from build123d import *

# Parameters (mm, degrees)
SKETCH_1_R      = 10
SKETCH_1_R_2    = 1.25
SKETCH_1_R_3    = 3
EXTRUDE_1_DEPTH = 2
SKETCH_2_R      = 4.5
SKETCH_2_R_2    = 3
EXTRUDE_2_DEPTH = 1


with BuildPart() as part:
    # 草图1 → 凸台-拉伸1 (new body)
    with BuildSketch(Plane.XY):
        Circle(SKETCH_1_R)
        with Locations((-4.949747468, 4.949747468)):
            Circle(SKETCH_1_R_2, mode=Mode.SUBTRACT)
        with Locations((4.949747468, 4.949747468)):
            Circle(SKETCH_1_R_2, mode=Mode.SUBTRACT)
        with Locations((4.949747468, -4.949747468)):
            Circle(SKETCH_1_R_2, mode=Mode.SUBTRACT)
        with Locations((-4.949747468, -4.949747468)):
            Circle(SKETCH_1_R_2, mode=Mode.SUBTRACT)
        Circle(SKETCH_1_R_3, mode=Mode.SUBTRACT)
    extrude(amount=EXTRUDE_1_DEPTH)

    # 草图2 → 凸台-拉伸2 (add)
    with BuildSketch(Plane.XY.offset(2)):
        Circle(SKETCH_2_R)
        Circle(SKETCH_2_R_2, mode=Mode.SUBTRACT)
    extrude(amount=EXTRUDE_2_DEPTH)


solid = part.part
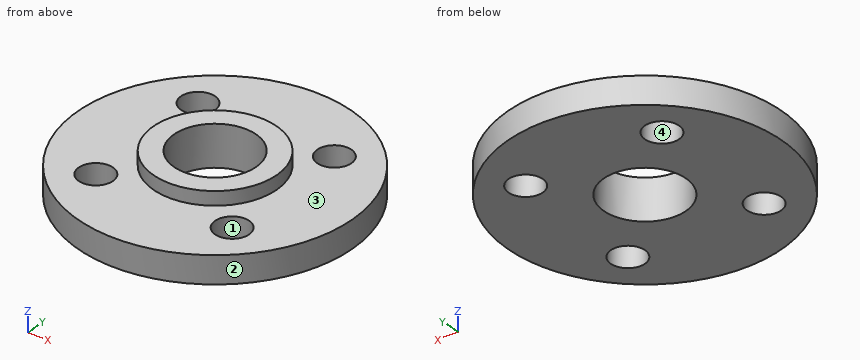
Check sheet for the modelled part. Datum: model origin and axes. Units: mm. Face numbers are marked on the shaded views. Round coordinates to 2 decimals unless told otherwise and drop trailing zeros. Loops run counter-clockwise (first coordinate to the right, second up) from the corner with the lowest first, then second, coordinate; pieces in that order, holes last. Notation, with made-up numbers: M 76,-36 L 85,-36 A19 ccw 85,-8 Z; hole C -20,-11.5 d2. An arc over 180 degrees is marked long. One line per item, written item: value.
(1) Sectioned sample at D-D, the plane z = 2.75. Record the cut outline in (x, y).
Computed values:
outline: C 0,0 d9; hole C 0,0 d6
(2) Release check for a two-part mould opening along X. For the marked faces 1, 2, 3 and 4 record: +X half, -X half, draft (parallel to the pull), parting line (faces both ways), or undercut.
Computed values:
face 1: undercut
face 2: parting line
face 3: draft
face 4: undercut
(3) Sectioned sample at A-A, the plane x = 0. Record the cut outline in (y, z).
Computed values:
outline: M -10,0 L -3,0 L -3,3 L -4.5,3 L -4.5,2 L -10,2 Z; M 3,0 L 10,0 L 10,2 L 4.5,2 L 4.5,3 L 3,3 Z
(4) Thickness scan on line 1 (Y direction, x = 0, z = 0.55); line 2 (X direction, y = -5.5, z = 1.3); line 3 (X direction, y = 5.75, z = 0.8). Record the ranges inside material, lowest first.
Computed values:
line 1: y = -10 to -3, 3 to 10
line 2: x = -8.35 to -6.07, -3.83 to 3.83, 6.07 to 8.35
line 3: x = -8.18 to -5.91, -3.99 to 3.99, 5.91 to 8.18
(5) Depth check by flat-ended pin: pin 1 Ø3 at (x, y) = (4.95, -4.95) entering from -Z; pin 2 Ø4 at (x, y) = (-4.95, -4.95) entering from +Z. Enter the tip coordinate at first touch or a pass-through.
Computed values:
pin 1: stops at z = 0
pin 2: stops at z = 2
(6) Sectioned sample at C-C, the plane y = 5.5. Record the cut outline in (x, z).
Computed values:
outline: M -8.35,0 L -6.07,0 L -6.07,2 L -8.35,2 Z; M -3.83,0 L 3.83,0 L 3.83,2 L -3.83,2 Z; M 6.07,0 L 8.35,0 L 8.35,2 L 6.07,2 Z
